from build123d import *

# Parameters (mm, degrees)
SKETCH_1_W          = 110
SKETCH_1_H          = 100
SKETCH_1_R          = 2.15
EXTRUDE_1_DEPTH     = 1
SKETCH_2_R          = 1.7
CUT_EXTRUDE_1_DEPTH = 15


with BuildPart() as part:
    # Эскиз1 → Бобышка-Вытянуть1 (new, symmetric)
    with BuildSketch(Plane.XY):
        Rectangle(SKETCH_1_W, SKETCH_1_H)
        with Locations((-50, 45)):
            Circle(SKETCH_1_R, mode=Mode.SUBTRACT)
        with Locations(Location((50, 45, 0), (0, 0, 180))):
            Circle(SKETCH_1_R, mode=Mode.SUBTRACT)
        with Locations((50, -45)):
            Circle(SKETCH_1_R, mode=Mode.SUBTRACT)
        with Locations(Location((-50, -45, 0), (0, 0, 180))):
            Circle(SKETCH_1_R, mode=Mode.SUBTRACT)
    extrude(amount=EXTRUDE_1_DEPTH, both=True)

    # Эскиз2 → Вырез-Вытянуть1 (cut)
    with BuildSketch(Plane.XY.offset(1)):
        with Locations((22, 19.85)):
            Circle(SKETCH_2_R)
        with Locations((-11.5, 19.85)):
            Circle(SKETCH_2_R)
        with Locations((22, -19.885932887)):
            Circle(SKETCH_2_R)
        with Locations((-11.5, -19.85)):
            Circle(SKETCH_2_R)
    extrude(amount=-CUT_EXTRUDE_1_DEPTH, mode=Mode.SUBTRACT)


solid = part.part
Read the model definition and answer for the solid it produces. Units are mm, in the model's axes. Coordinates: 2 decimals unless noted, no trailing zeros. Order: outer loops, then holes, each group sorted by start corner. A loop starts at its lowest first (then second) coordinate and runs counter-clockwise, first axis right, second up. Notation, with made-up numbers: M 55,-29 L 84,-29 A13 ccw 84,-5 Z; hole C 87.25,78 d4. An arc over 180 degrees is marked long. Put each result on its own line as item: value. Start each with the question number.
Item 1: Section A-A, the plane x = 22 is taken. Determine the outline of the cut face in (y, z).
Item 2: Given pin 1 Ø2.5 at (x, y) = (-50, 45) entering from -Z, flat-ended and moving along its own axis, determine where the tip first touches the part or whether it passes through.
Item 3: The mould has two halves that part along X. Classify faces 1 (the face through (-1, 1, 1)), 2 (the face through (48.84, 43.19, -0.01)), 3 (the face through (-51.16, -46.81, -0.01)): +X half, -X half, draft (parallel to the pull), parting line (faces both ways), or undercut.
Item 4: Consider probe 1 along Y at (x, z) = (-50, -0.15); probe 2 along Y at (x, z) = (-11.5, 0.5); probe 3 along X at (y, z) = (-21, -0.1). Determine where each line is inside the solid, lowest interval first. Write a range as [from, to].
Item 5: Section B-B, the plane y = 19.85 is taken. Determine the outline of the cut face in (x, z), plus the area to 3 significant figures.
Computed:
1. outline: M -50,-1 L -21.59,-1 L -21.59,1 L -50,1 Z; M -18.19,-1 L 18.15,-1 L 18.15,1 L -18.19,1 Z; M 21.55,-1 L 50,-1 L 50,1 L 21.55,1 Z
2. pin 1: passes through
3. face 1: draft
3. face 2: undercut
3. face 3: undercut
4. probe 1: y = [-50, -47.15], [-42.85, 42.85], [47.15, 50]
4. probe 2: y = [-50, -21.55], [-18.15, 18.15], [21.55, 50]
4. probe 3: x = [-55, -12.75], [-10.25, 20.72], [23.28, 55]
5. outline: M -55,-1 L -13.2,-1 L -13.2,1 L -55,1 Z; M -9.8,-1 L 20.3,-1 L 20.3,1 L -9.8,1 Z; M 23.7,-1 L 55,-1 L 55,1 L 23.7,1 Z
5. area: 206 mm2
